from build123d import *

# Parameters (mm, degrees)
SKETCH1_R           = 1.6
BOSS_EXTRUDE1_DEPTH = 8
CHAMFER1_SIZE       = 1


with BuildPart() as part:
    # Sketch1 → Boss-Extrude1 (new body)
    with BuildSketch(Plane.XY):
        with BuildLine():
            Line((-0.5, 3), (105.5, 3))
            ThreePointArc((105.5, 3), (107.267766953, 2.267766953), (108, 0.5))
            Line((108, 0.5), (108, -0.5))
            ThreePointArc((108, -0.5), (107.267766953, -2.267766953), (105.5, -3))
            Line((105.5, -3), (-0.5, -3))
            ThreePointArc((-0.5, -3), (-2.267766953, -2.267766953), (-3, -0.5))
            Line((-3, -0.5), (-3, 0.5))
            ThreePointArc((-3, 0.5), (-2.267766953, 2.267766953), (-0.5, 3))
        make_face()
        Circle(SKETCH1_R, mode=Mode.SUBTRACT)
        with Locations((7.5, 0)):
            Circle(SKETCH1_R, mode=Mode.SUBTRACT)
        with Locations((15, 0)):
            Circle(SKETCH1_R, mode=Mode.SUBTRACT)
        with Locations((22.5, 0)):
            Circle(SKETCH1_R, mode=Mode.SUBTRACT)
        with Locations((30, 0)):
            Circle(SKETCH1_R, mode=Mode.SUBTRACT)
        with Locations((37.5, 0)):
            Circle(SKETCH1_R, mode=Mode.SUBTRACT)
        with Locations((45, 0)):
            Circle(SKETCH1_R, mode=Mode.SUBTRACT)
        with Locations((52.5, 0)):
            Circle(SKETCH1_R, mode=Mode.SUBTRACT)
        with Locations((60, 0)):
            Circle(SKETCH1_R, mode=Mode.SUBTRACT)
        with Locations((67.5, 0)):
            Circle(SKETCH1_R, mode=Mode.SUBTRACT)
        with Locations((75, 0)):
            Circle(SKETCH1_R, mode=Mode.SUBTRACT)
        with Locations((82.5, 0)):
            Circle(SKETCH1_R, mode=Mode.SUBTRACT)
        with Locations((90, 0)):
            Circle(SKETCH1_R, mode=Mode.SUBTRACT)
        with Locations((97.5, 0)):
            Circle(SKETCH1_R, mode=Mode.SUBTRACT)
        with Locations((105, 0)):
            Circle(SKETCH1_R, mode=Mode.SUBTRACT)
    extrude(amount=BOSS_EXTRUDE1_DEPTH)

    # Chamfer1
    chamfer1_edges = [part.edges().sort_by_distance(p)[0] for p in [
        (-1.6, 0, 0),
        (-1.6, 0, 8),
        (5.9, 0, 0),
        (5.9, 0, 8),
        (13.4, 0, 0),
        (13.4, 0, 8),
        (20.9, 0, 0),
        (20.9, 0, 8),
        (28.4, 0, 0),
        (28.4, 0, 8),
        (35.9, 0, 0),
        (35.9, 0, 8),
        (43.4, 0, 0),
        (43.4, 0, 8),
        (50.9, 0, 0),
        (50.9, 0, 8),
        (58.4, 0, 0),
        (58.4, 0, 8),
        (65.9, 0, 0),
        (65.9, 0, 8),
        (73.4, 0, 0),
        (73.4, 0, 8),
        (80.9, 0, 0),
        (80.9, 0, 8),
        (88.4, 0, 0),
        (88.4, 0, 8),
        (95.9, 0, 0),
        (95.9, 0, 8),
        (103.4, 0, 0),
        (103.4, 0, 8),
    ]]
    chamfer(chamfer1_edges, length=CHAMFER1_SIZE)


solid = part.part
Here's how the part is built. I have some questions about the finished solid (model axes, mm). Round coordinates to 2 decimals unless told otherwise and drop trailing zeros. Loops run counter-clockwise (first coordinate to the right, second up) from the corner with the lowest first, then second, coordinate; pieces in that order, holes last. Notation, with made-up numbers: (13.5, 56.25) - (53.5, 56.25) arc R25 cw to (53.5, 81.25) - close; hole circle Ø7 at (-7, 79). An arc over 180 degrees is marked (long way). One line per question, with ' | ' between items. Start each with the question number.
Q1. I want a section at A-A (x = 75). Write out the boundary of the cut face in (y, z), then the cut area to 3 significant figures.
Q2. I want a section at B-B (z = 5.5). State how many separate pieces and enclosed holes the cut face has, then the cut area to 3 significant figures.
Q3. Please list where these lines run through material, in increasing order: line 1 (Y direction, x = 60, z = 2.6); line 2 (X direction, y = -1.85, z = 6.25); line 3 (Y direction, x = 31, z = 3). Write a range as [from, to].
Q4. We'd pull the mould along X, two halves only. Please class faces 1 (the cylindrical face through (69.026, 0.481, 3.958)), 2 (the cylindrical face through (-2.248, -2.287, 3.944)): +X half, -X half, draft (parallel to the pull), parting line (faces both ways), or undercut.
Q5. Will these pins go through, and if not, where does the flat tip stop? pin 1 (3.5 mm diameter, centred on x = 30, y = 0, fed in from -Z); pin 2 (1.9 mm diameter, centred on x = 52.5, y = 0, fed in from +Z); pin 3 (3.5 mm diameter, centred on x = 0, y = 0, fed in from +Z); pin 4 (2 mm diameter, centred on y = 2, z = 4, fed in from -X).
Response values:
1) outline: (-3, 0) - (-2.6, 0) - (-1.6, 1) - (-1.6, 7) - (-2.6, 8) - (-3, 8) - close; (1.6, 1) - (2.6, 0) - (3, 0) - (3, 8) - (2.6, 8) - (1.6, 7) - close | area: 20.4 mm²
2) separate pieces: 1 | enclosed holes: 15 | area: 540 mm²
3) line 1: y = [-3, -1.6], [1.6, 3] | line 2: x = [-2.6, 107.6] | line 3: y = [-3, -1.25], [1.25, 3]
4) face 1: undercut | face 2: -X half
5) pin 1: stops at z = 0.85 | pin 2: passes through | pin 3: stops at z = 7.15 | pin 4: stops at x = -2.95
